Input: part model. Units: mm. Frame: model coordinates. Give positions to 0.01 mm unless a question says otherwise; leave off trailing zeros. Loops run counter-clockwise (first coordinate to the right, second up) from the corner with the lowest first, then second, coordinate; pieces in that order, holes last. Notation, with made-up numbers: M 69,12 L 75,12 A16 ccw 75,25 Z; hole C -22.75,80 d8. An arc over 180 degrees is marked long. Answer as a JSON object with one key per item and string values. Group by question number.
1) Section query A-A on x = 62.5. Return loops of the section in (y, z), plus the area to 3 significant figures.
2) Ray query, L1, parallel to X at y = 1.2, z = -30; L2, parallel to Z at x = 62.5, y = 1.25. Return the intervals inside material, ascending.
3) Section query B-B on z = -30. Return loops of the section in (x, y).
from build123d import *

# Parameters (mm, degrees)
SKETCH1_W                      = 135
SKETCH1_H                      = 70
BOSS_EXTRUDE1_DEPTH            = 1.6
CUT_EXTRUDE1_REACH             = 78.051
SKETCH2_R                      = 1.5
CUT_EXTRUDE1_DIRECTION_2_DEPTH = 77.051364222


with BuildPart() as part:
    # Sketch1 → Boss-Extrude1 (new body)
    with BuildSketch(Plane(origin=(0, 0, 0), x_dir=(1, 0, 0), z_dir=(0, 1, 0))):
        Rectangle(SKETCH1_W, SKETCH1_H)
    extrude(amount=BOSS_EXTRUDE1_DEPTH)

    # Sketch2 → Cut-Extrude1 (cut, up to next)
    with BuildSketch(Plane(origin=(0, 1.6, 0), x_dir=(1, 0, 0), z_dir=(0, 1, 0)), mode=Mode.PRIVATE) as cut_extrude1_sk1:
        with Locations(Location((-62.5, 30, 0), (0, 0, 90))):
            Circle(SKETCH2_R)
    cut_extrude1_tool1 = extrude(cut_extrude1_sk1.sketch, amount=-CUT_EXTRUDE1_REACH, mode=Mode.PRIVATE) & part.part
    # Sketch2 → Cut-Extrude1 (cut, up to next)
    with BuildSketch(Plane(origin=(0, 1.6, 0), x_dir=(1, 0, 0), z_dir=(0, 1, 0)), mode=Mode.PRIVATE) as cut_extrude1_sk2:
        with Locations(Location((62.5, 30, 0), (0, 0, 90))):
            Circle(SKETCH2_R)
    cut_extrude1_tool2 = extrude(cut_extrude1_sk2.sketch, amount=-CUT_EXTRUDE1_REACH, mode=Mode.PRIVATE) & part.part
    # Sketch2 → Cut-Extrude1 (cut, up to next)
    with BuildSketch(Plane(origin=(0, 1.6, 0), x_dir=(1, 0, 0), z_dir=(0, 1, 0)), mode=Mode.PRIVATE) as cut_extrude1_sk3:
        with Locations(Location((62.5, -30, 0), (0, 0, 90))):
            Circle(SKETCH2_R)
    cut_extrude1_tool3 = extrude(cut_extrude1_sk3.sketch, amount=-CUT_EXTRUDE1_REACH, mode=Mode.PRIVATE) & part.part
    # Sketch2 → Cut-Extrude1 (cut, up to next)
    with BuildSketch(Plane(origin=(0, 1.6, 0), x_dir=(1, 0, 0), z_dir=(0, 1, 0)), mode=Mode.PRIVATE) as cut_extrude1_sk4:
        with Locations(Location((-62.5, -30, 0), (0, 0, 90))):
            Circle(SKETCH2_R)
    cut_extrude1_tool4 = extrude(cut_extrude1_sk4.sketch, amount=-CUT_EXTRUDE1_REACH, mode=Mode.PRIVATE) & part.part
    add(cut_extrude1_tool1.solids().sort_by_distance((-62.5, 1.6, -30))[0], mode=Mode.SUBTRACT)
    add(cut_extrude1_tool2.solids().sort_by_distance((62.5, 1.6, -30))[0], mode=Mode.SUBTRACT)
    add(cut_extrude1_tool3.solids().sort_by_distance((62.5, 1.6, 30))[0], mode=Mode.SUBTRACT)
    add(cut_extrude1_tool4.solids().sort_by_distance((-62.5, 1.6, 30))[0], mode=Mode.SUBTRACT)

    # Sketch2 → Cut-Extrude1 direction 2 (cut)
    with BuildSketch(Plane(origin=(0, 1.6, 0), x_dir=(1, 0, 0), z_dir=(0, 1, 0))):
        with Locations(Location((-62.5, 30, 0), (0, 0, 90))):
            Circle(SKETCH2_R)
        with Locations(Location((62.5, 30, 0), (0, 0, 90))):
            Circle(SKETCH2_R)
        with Locations(Location((62.5, -30, 0), (0, 0, 90))):
            Circle(SKETCH2_R)
        with Locations(Location((-62.5, -30, 0), (0, 0, 90))):
            Circle(SKETCH2_R)
    extrude(amount=CUT_EXTRUDE1_DIRECTION_2_DEPTH, mode=Mode.SUBTRACT)


solid = part.part
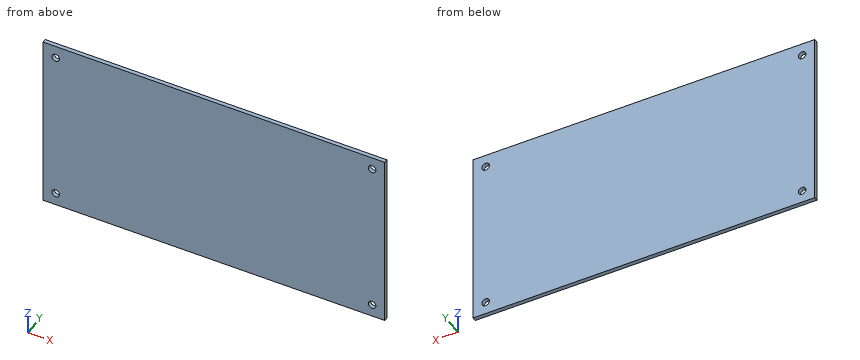
Output:
{
 "1": {"outline": "M 0,-35 L 1.6,-35 L 1.6,-31.5 L 0,-31.5 Z; M 0,-28.5 L 1.6,-28.5 L 1.6,28.5 L 0,28.5 Z; M 0,31.5 L 1.6,31.5 L 1.6,35 L 0,35 Z", "area": "102 mm^2"},
 "2": {"L1": "x = -67.5 to -64, -61 to 61, 64 to 67.5", "L2": "z = -35 to -31.5, -28.5 to 28.5, 31.5 to 35"},
 "3": {"outline": "M -67.5,0 L -64,0 L -64,1.6 L -67.5,1.6 Z; M -61,0 L 61,0 L 61,1.6 L -61,1.6 Z; M 64,0 L 67.5,0 L 67.5,1.6 L 64,1.6 Z"}
}
